Could you check a few things on this model? Use its own coordinates, in mm. A direction names the side the tool comes from. Give positions to 0.01 mm unless a question says otherwise; leave off trailing zeros. Order: outer loops, then holes, each group sorted by start corner. A loop starts at its lowest first (then second) coordinate and runs counter-clockwise, first axis right, second up. Notation, with made-up numbers: (57, 77) -> (100, 77) arc R8 cw to (100, 88) -> close; hole circle Ø5 at (82, -7). An arc over 180 degrees is marked (long way). One line per item, written item: value.
```python
from build123d import *

# Parameters (mm, degrees)
F0_R     = 46.303997109
F1_DEPTH = 6.35
F0_R_2   = 50.7773250867
F2_DEPTH = 12.7
F5_DEPTH = 6.35


# Not quite as in the source:
# - a fillet or chamfer that OpenCascade refuses, or shapes differently, is made with other operations: its cross-section is extruded or revolved along the edge and cut away or added


with BuildPart() as f1:
    # F0 (on Top) → F1 (new body)
    with BuildSketch(Plane.XY):
        Circle(F0_R)
    extrude(amount=F1_DEPTH)

    # F0 (on Top) → F2 (join)
    with BuildSketch(Plane.XY):
        Circle(F0_R_2)
        Circle(F0_R, mode=Mode.SUBTRACT)
    extrude(amount=F2_DEPTH)

    # F3: fillet of radius 5.08 on 1 edges, made by hand

    # F3_s1 → F3_t2 (revolve, cut)
    with BuildSketch(Plane.XZ):
        with BuildLine():
            ThreePointArc((50.7773250867, 7.6563555778), (49.4978706971, 11.0271497073), (46.303997109, 12.7))
            Line((46.303997109, 12.7), (46.3161305494, 12.8008728884))
            ThreePointArc((46.3161305494, 12.8008728884), (48.5406610978, 12.8016), (50.7773250867, 12.8016))
            Line((50.7773250867, 12.8016), (50.8789250867, 12.7))
            Line((50.8789250867, 12.7), (50.8789250867, 7.6563555778))
            Line((50.8789250867, 7.6563555778), (50.7773250867, 7.6563555778))
        make_face()
    revolve(axis=Axis((0, 0, 12.7), (0, 0, 1)), mode=Mode.SUBTRACT)

    # F4 (on face) → F5 (join)
    with BuildSketch(Plane.XY.offset(6.35)):
        Polygon((-8.1779062748, -15.8028278183), (-26.3735784938, -55.8334334653), (14.7386826575, -3.0078946147), (5.1134219393, -3.0078946147), (20.4086864271, 16.6451374931), (10.8284205198, 16.6451374931), (28.2742083073, 59.8571076989), (-8.1779062748, 5.9409798123), (2.4016224779, 9.0941041708), (-16.5434218943, -20.15289478), align=None)
    extrude(amount=F5_DEPTH)


solid = f1.part
```
1) For faces 1 (the flat face through (-6.938, -5.325, 9.481)), 2 (the flat face through (24, 51, 6.35)), 3 (the flat face through (-1, 1, 0)), which set-ups out of +Z, -Z, +X, -X, +Y, -Y let a thin tool reach every point of the face, with its end or its side?
Answer below:
face 1: +Z
face 2: -Z, +X, +Y
face 3: -Z, +X, -X, +Y, -Y
2) We'd pull the mould along X, two halves only. Please class faces 4 (the flat face through (-1.135, -23.404, 9.481)), 5 (the flat face through (25.32, 52.54, 9.48)), 6 (the flat face through (-23, -50, 6.35)), 7 (the flat face through (-23.843, -50.266, 9.481)): +X half, -X half, draft (parallel to the pull), parting line (faces both ways), or undercut.
Answer below:
face 4: undercut
face 5: +X half
face 6: draft
face 7: -X half
3) For P1, Ø5.5, axis at x = -22, y = -53, coming from the -Z side; P2, Ø1.9, axis at x = 7.5, z = 8.5, coming from the +Y side; P3, Ø1, axis at x = -31.5, z = 3, coming from the -Y side, each with a flat end and sliding along its axis, tell me the tip position at first contact or that it passes through.
Answer below:
P1: stops at z = 6.35
P2: stops at y = 50.32
P3: stops at y = -40.22
4) Suppose I cut it at D-D, the plane z = 3.75. Write out the boundary of the cut face in (x, y).
Answer below:
outline: circle Ø101.55 at (0, 0)
5) If I drill on line 1 along X through (y, z) = (17.5, 8.75); line 2 along X through (y, z) = (4.5, 9.75); line 3 along Y through (x, z) = (-25.5, 11.5), over which ranges is the centre line in solid material (lowest first)?
Answer below:
line 1: x = -47.54 to -42.87, -0.36 to 11.17, 42.87 to 47.54
line 2: x = -50.12 to -46.08, -0.57 to 10.96, 46.08 to 50.12
line 3: y = -54.71 to -53.91, -41.86 to -38.65, 38.65 to 41.86
6) Suppose I cut it at C-C, the plane y = 0. Write out the boundary of the cut face in (x, z).
Answer below:
outline: (-50.78, 0) -> (50.78, 0) -> (50.78, 7.66) arc R5.08 ccw to (46.3, 12.7) -> (46.3, 6.35) -> (7.45, 6.35) -> (7.45, 12.7) -> (-3.49, 12.7) -> (-3.49, 6.35) -> (-46.3, 6.35) -> (-46.3, 12.7) arc R5.08 ccw to (-50.78, 7.66) -> close
7) Suppose I cut it at B-B, the plane x = 0. Write out the boundary of the cut face in (y, z), then the cut area to 3 significant figures.
Answer below:
outline: (-50.78, 0) -> (50.78, 0) -> (50.78, 7.66) arc R5.08 ccw to (46.3, 12.7) -> (46.3, 6.35) -> (18.04, 6.35) -> (18.04, 12.7) -> (8.38, 12.7) -> (8.38, 6.35) -> (5.39, 6.35) -> (5.39, 12.7) -> (-21.95, 12.7) -> (-21.95, 6.35) -> (-46.3, 6.35) -> (-46.3, 12.7) arc R5.08 ccw to (-50.78, 7.66) -> close
area: 926 mm2
